```python
from build123d import *

# Parameters (mm, degrees)
SKETCH1_W           = 430
SKETCH1_H           = 450
BOSS_EXTRUDE1_DEPTH = 8
SKETCH2_W           = 175
SKETCH2_H           = 100
CUT_EXTRUDE1_DEPTH  = 10
SKETCH4_R           = 3.5
BOSS_EXTRUDE3_DEPTH = 15
BOSS_EXTRUDE4_DEPTH = 90
SKETCH9_W           = 430
SKETCH9_H           = 5
BOSS_EXTRUDE6_DEPTH = 7.5
SKETCH10_W          = 430
SKETCH10_H          = 20
BOSS_EXTRUDE7_DEPTH = 2.5


with BuildPart() as part:
    # Sketch1 → Boss-Extrude1 (new body)
    with BuildSketch(Plane(origin=(0, 0, 0), x_dir=(1, 0, 0), z_dir=(0, 1, 0))):
        with Locations((215, 225)):
            Rectangle(SKETCH1_W, SKETCH1_H)
    extrude(amount=BOSS_EXTRUDE1_DEPTH)

    # Sketch2 → Cut-Extrude1 (cut)
    with BuildSketch(Plane(origin=(0, 8, 0), x_dir=(1, 0, 0), z_dir=(0, 1, 0))):
        with Locations((215, 50)):
            Rectangle(SKETCH2_W, SKETCH2_H)
    extrude(amount=-CUT_EXTRUDE1_DEPTH, mode=Mode.SUBTRACT)

    # Sketch4 → Boss-Extrude3 (add)
    with BuildSketch(Plane.XZ):
        with Locations((30, -217)):
            Circle(SKETCH4_R)
        with Locations((400, -217)):
            Circle(SKETCH4_R)
    extrude(amount=BOSS_EXTRUDE3_DEPTH)

    # Sketch5 → Boss-Extrude4 (add)
    with BuildSketch(Plane.XZ):
        Polygon((5.000626144, -445), (0, -445), (0, -450), (430, -450), (430, -445), (429.008283612, -445), align=None)
    extrude(amount=BOSS_EXTRUDE4_DEPTH)

    # Sketch9 → Boss-Extrude6 (add)
    with BuildSketch(Plane.XZ):
        with Locations((215, -370)):
            Rectangle(SKETCH9_W, SKETCH9_H)
    boss_extrude6 = extrude(amount=BOSS_EXTRUDE6_DEPTH)

    # Sketch10 → Boss-Extrude7 (add)
    with BuildSketch(Plane.XZ.offset(7.5)):
        with Locations((215, -370)):
            Rectangle(SKETCH10_W, SKETCH10_H)
    boss_extrude7 = extrude(amount=BOSS_EXTRUDE7_DEPTH)

    # Mirror9: Boss-Extrude6, Boss-Extrude7 across plane
    add(boss_extrude6.mirror(Plane.XY.offset(-315)))
    add(boss_extrude7.mirror(Plane.XY.offset(-315)))


solid = part.part
```
For this review, take the finished solid that the model builds, in its own axes (mm). A direction names the side the tool comes from. Give positions to 0.01 mm unless a question says otherwise; leave off trailing zeros. Write each loop counter-clockwise with the first axis right and the second up, starting at its lowest first coordinate (ties: lowest second). Pieces come first, ordered by that corner, then holes. Notation, with made-up numbers: M 3,3 L 46,3 A17 cw 46,14 Z; hole C -38.75,-13.5 d9. An arc over 180 degrees is marked long. One line per item, written item: value.
1) Take a section at D-D, the plane y = -74. Write out the cut boundary in (x, z), then the cut area to 3 significant figures.
Results are:
outline: M 0,-450 L 430,-450 L 430,-445 L 0,-445 Z
area: 2,150 mm²
2) For line 1 (Y direction, x = 364, z = -252.5); line 2 (Z direction, x = 280, y = -39); line 3 (Y direction, x = 365, z = -208.5), list the stretches that pass through material, from the lowest coordinate up. Write a range as from..to.
Results are:
line 1: y = -10..-7.5, 0..8
line 2: z = -450..-445
line 3: y = 0..8
3) Take a section at C-C, the plane z = -130.5. Write out the cut boundary in (x, y).
Results are:
outline: M 0,0 L 430,0 L 430,8 L 0,8 Z
4) The part is to be moulded in two halves that separate along Z. For faces 1 (the flat face through (212, -40, -450)), 2 (the flat face through (0, 3, -224)), 3 (the flat face through (212, 0, -316)), say which applies: +Z half, -Z half, draft (parallel to the pull), parting line (faces both ways), or undercut.
Results are:
face 1: -Z half
face 2: draft
face 3: undercut
5) For P1, Ø7.5, axis at x = 398.5, z = -216.5, coming from the -Y side; P2, Ø1.5, axis at x = 381.5, z = -176, coming from the -Y side; P3, Ø2, axis at x = 263.5, y = -2.5, coming from the +Z side; P4, Ø4, axis at y = 2.5, z = -63.5, coming from the -X side, all flat-tipped, find the tip position at first contact; note any pin that passes through.
Results are:
P1: stops at y = -15
P2: stops at y = 0
P3: stops at z = -257.5
P4: stops at x = 0
6) Take a section at B-B, the plane x = 53. Write out the cut boundary in (y, z), then the cut area to 4 significant figures.
Results are:
outline: M -90,-450 L 8,-450 L 8,0 L 0,0 L 0,-257.5 L -7.5,-257.5 L -7.5,-250 L -10,-250 L -10,-270 L -7.5,-270 L -7.5,-262.5 L 0,-262.5 L 0,-367.5 L -7.5,-367.5 L -7.5,-360 L -10,-360 L -10,-380 L -7.5,-380 L -7.5,-372.5 L 0,-372.5 L 0,-445 L -90,-445 Z
area: 4,225 mm²
7) Take a section at A-A, the plane z = -43. Write out the cut boundary in (x, y).
Results are:
outline: M 0,0 L 127.5,0 L 127.5,8 L 0,8 Z; M 302.5,0 L 430,0 L 430,8 L 302.5,8 Z
8) For faces 4 (the flat face through (218, -44, -445)), 5 (the flat face through (430, 3, -224)), list the 3-axis set-ups (+Z, -Z, +X, -X, +Y, -Y) from which the entire face can be reached by the end or side of a thin tool; tool diameter is ignored.
Results are:
face 4: +X, -X, -Y
face 5: +Z, -Z, +X, +Y, -Y
